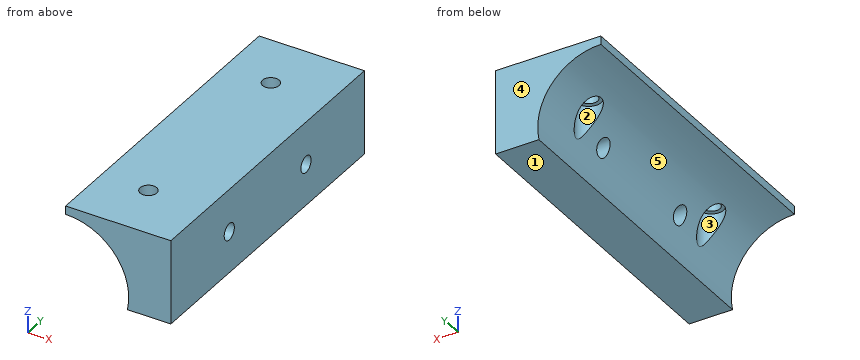
```python
from build123d import *

# Parameters (mm, degrees)
F0_W     = 25.4
F0_H     = 20.32
F1_DEPTH = 76.2
F2_R     = 15.24
F3_DEPTH = 76.2
F4_R     = 2
F5_DEPTH = 25
F6_R     = 3
F7_DEPTH = 16.5
F8_R     = 2
F9_DEPTH = 25


with BuildPart() as f1:
    # F0 (on Front) → F1 (new body)
    with BuildSketch(Plane.XZ):
        with Locations((12.7, 10.16)):
            Rectangle(F0_W, F0_H)
    extrude(amount=F1_DEPTH)

    # F2 (on face) → F3 (cut)
    with BuildSketch(Plane.XZ.offset(76.2)):
        with Locations((0, 3.048)):
            Circle(F2_R)
    extrude(amount=-F3_DEPTH, mode=Mode.SUBTRACT)

    # F4 (on face) → F5 (cut)
    with BuildSketch(Plane.XY.offset(20.32)):
        with Locations((11.4, -14)):
            Circle(F4_R)
        with Locations((11.4, -62.2)):
            Circle(F4_R)
    extrude(amount=-F5_DEPTH, mode=Mode.SUBTRACT)

    # F6 (on Top) → F7 (cut)
    with BuildSketch(Plane.XY):
        with Locations((11.5, -14)):
            Circle(F6_R)
        with Locations((11.5, -62.20332)):
            Circle(F6_R)
    extrude(amount=F7_DEPTH, mode=Mode.SUBTRACT)

    # F8 (on face) → F9 (cut)
    with BuildSketch(Plane.YZ.offset(25.4)):
        with Locations((-23, 10)):
            Circle(F8_R)
        with Locations((-53.2, 10)):
            Circle(F8_R)
    extrude(amount=-F9_DEPTH, mode=Mode.SUBTRACT)


solid = f1.part
```
Check sheet for the modelled part. Datum: model origin and axes. Units: mm. Face numbers are marked on the shaded views. A direction names the side the tool comes from. Give positions to 0.01 mm unless a question says otherwise; leave off trailing zeros. Write each loop counter-clockwise with the first axis right and the second up, starting at its lowest first coordinate (ties: lowest second). Pieces come first, ordered by that corner, then holes. Notation, with made-up numbers: (12.25, 64.25) - (42.25, 64.25) arc R22 cw to (42.25, 98.25) - close; hole circle Ø3 at (-19, 11). An arc over 180 degrees is marked (long way). Answer as a JSON object with one key per item and string values. Group by question number.
1) Release check for a two-part mould opening along X. For the marked faces 3, 4 and 5 record: pulls with the +X half, pulls with the -X half, needs draft (parallel to the pull), parting line crosses it, or undercut.
2) Sectioned sample at D-D (x = 11.4). Record the cut outline in (y, z), then the cut area to 3 significant figures.
3) Sectioned sample at C-C (z = 10). Record the cut outline in (x, y).
4) Depth check by flat-ended pin: P1, Ø3, axis at x = 12, y = -61, coming from the -Z side; P2, Ø10, axis at y = -30.5, z = 10, coming from the -X side; P3, Ø10, axis at x = 7, y = -33, coming from the -Z side. Enter the tip coordinate at first touch or a pass-through.
5) Sectioned sample at B-B (y = -14). Record the cut outline in (x, z), then the cut area to 3 significant figures.
6) Thickness scan on probe 1 along Y at (x, z) = (15.5, 10); probe 2 along Y at (x, z) = (11.4, 17.8); probe 3 along Z at (x, y) = (22, -53.2). Record the ranges inside material, lowest first. Write a range as from..to.
7) Access from +Z, -Z, +X, -X, +Y, -Y to the whole of each face (thin tool, end or side, straight path). Record for the marked faces 1 and 2.
8) Sectioned sample at A-A (x = 23.5). Record the cut outline in (y, z), then the cut area to 3 significant figures.
Geometry results:
{
 "1": {"face 3": "undercut", "face 4": "needs draft", "face 5": "pulls with the -X half"},
 "2": {"outline": "(-76.2, 13.16) - (-65.2, 13.16) - (-65.2, 16.5) - (-64.2, 16.5) - (-64.2, 20.32) - (-76.2, 20.32) - close; (-60.2, 16.5) - (-59.2, 16.5) - (-59.2, 13.16) - (-17, 13.16) - (-17, 16.5) - (-16, 16.5) - (-16, 20.32) - (-60.2, 20.32) - close; (-12, 16.5) - (-11, 16.5) - (-11, 13.16) - (0, 13.16) - (0, 20.32) - (-12, 20.32) - close", "area": "475 mm^2"},
 "3": {"outline": "(13.56, -76.2) - (25.4, -76.2) - (25.4, -55.2) - (13.56, -55.2) - (13.56, -60.02) arc R3 cw to (13.56, -64.38) - close; (13.56, -51.2) - (25.4, -51.2) - (25.4, -25) - (13.56, -25) - close; (13.56, -21) - (25.4, -21) - (25.4, 0) - (13.56, 0) - (13.56, -11.82) arc R3 cw to (13.56, -16.18) - close"},
 "4": {"P1": "stops at z = 16.5", "P2": "stops at x = 9.46", "P3": "stops at z = 12.44"},
 "5": {"outline": "(0, 18.29) arc R15.24 cw to (8.5, 15.7) - (8.5, 16.5) - (9.4, 16.5) - (9.4, 20.32) - (0, 20.32) - close; (13.4, 16.5) - (14.5, 16.5) - (14.5, 7.74) arc R15.24 cw to (14.93, 0) - (25.4, 0) - (25.4, 20.32) - (13.4, 20.32) - close", "area": "249 mm^2"},
 "6": {"probe 1": "y = -76.2..-55.2, -51.2..-25, -21..0", "probe 2": "y = -76.2..-64.2, -60.2..-16, -12..0", "probe 3": "z = 0..8, 12..20.32"},
 "7": {"face 1": "-Z, +X, -X, +Y, -Y", "face 2": "-Z"},
 "8": {"outline": "(-76.2, 0) - (0, 0) - (0, 20.32) - (-76.2, 20.32) - close; hole circle Ø4 at (-53.2, 10); hole circle Ø4 at (-23, 10)", "area": "1,520 mm^2"}
}
